Here's how the part is built. I have some questions about the finished solid (model axes, mm). A direction names the side the tool comes from. Coordinates: 2 decimals unless noted, no trailing zeros. Loops run counter-clockwise (first coordinate to the right, second up) from the corner with the lowest first, then second, coordinate; pieces in that order, holes last. Notation, with made-up numbers: M 58,53 L 65,53 A18 cw 65,76 Z; hole C 22,84 d4. An arc over 180 degrees is marked long. Use one line per item in the form item = value. Start each with the question number.
(1) On a 3-axis mill with a long thin cutter (end or side, diameter ignored), from which of +Z, -Z, +X, -X, +Y, -Y can I reach the whole of each face in a straight line? I mean faces 5 (the flat face through (2.87, -3, 5)), 6 (the flat face through (0, 0, 22)). Say none if no direction works.
(2) Imagine slicing it at C-C, the plane z = 30.5. Please give me the cut outline in (x, y), and give its area (3 significant figures).
(3) Thinking about a two-plate mould opening in Z: for faces 1 (the flat face through (0, -2, 45)), 2 (the flat face through (1.455, -2.837, 7.788)), 3 (the flat face through (0, -2, 0)), 4 (the flat face through (5.44, -1, 22)), which applies, +Z half, -Z half, draft (parallel to the pull), parting line (faces both ways), or undercut?
(4) Imagine slicing it at D-D, the plane x = 2. Please give me the cut outline in (y, z), and give its area (3 significant figures).
(5) Will these pins go through, and if not, where does the flat tip stop? P1, Ø1.9, axis at y = -3, z = 4.5, coming from the -X side; P2, Ø3, axis at x = -1, z = 5, coming from the -Y side; P3, Ø1.9, axis at y = -3, z = 40, coming from the +X side; P4, Ø1, axis at x = -1.5, y = -0.5, coming from the -Z side.
(6) Imagine slicing it at B-B, the plane y = -2.4. Please give me the cut outline in (x, z), and give its area (3 significant figures).
(7) Imagine slicing it at A-A, the plane x = -0.5. Please give me the cut outline in (y, z), and give its area (3 significant figures).
(8) Please list where these lines run through material, in increasing order: L1, parallel to Z at x = 0, y = -0.4; L2, parallel to Z at x = 1, y = -1.5 (3 decimals); L3, parallel to Y at x = 2, z = 39.
```python
from build123d import *

# Parameters (mm, degrees)
PAD_DEPTH       = 45
SKETCH001_R     = 1.6
POCKET_DEPTH    = 4.001
POCKET001_DEPTH = 2.36


with BuildPart() as part:
    # Sketch → Pad (new body)
    with BuildSketch(Plane.XY):
        Polygon((0, 0), (-5.44, 0), (-5.44, -1.68), (-2.94, -4), (0, -4), (2.94, -4), (5.44, -1.68), (5.44, 0), align=None)
    extrude(amount=PAD_DEPTH)

    # Sketch001 (on Face5 of Pad) → Pocket (cut, through all)
    with BuildSketch(Plane.XZ.offset(4)):
        with Locations((0, 39.686009)):
            Circle(SKETCH001_R)
        with Locations((0, 5.313991)):
            Circle(SKETCH001_R)
    extrude(amount=-POCKET_DEPTH, mode=Mode.SUBTRACT)

    # Sketch002 (on Face10 of Pocket) → Pocket001 (cut)
    with BuildSketch(Plane.XZ.offset(4)):
        Polygon((2.87, 41.343005), (0, 43), (-2.87, 41.343005), (-2.87, 38.029014), (0, 36.372019), (2.87, 38.029014), align=None)
        Polygon((2.87, 6.970986), (0, 8.627981), (-2.87, 6.970986), (-2.87, 3.656995), (0, 2), (2.87, 3.656995), align=None)
    extrude(amount=-POCKET001_DEPTH, mode=Mode.SUBTRACT)


solid = part.part
```
Answer:
q1.face_5 = -Y
q1.face_6 = +Z, -Z, +X, -X, +Y
q2.outline = M -5.44,-1.68 L -2.94,-4 L 2.94,-4 L 5.44,-1.68 L 5.44,0 L -5.44,0 Z
q2.area = 37.7 mm²
q3.face_1 = +Z half
q3.face_2 = undercut
q3.face_3 = -Z half
q3.face_4 = draft
q4.outline = M -4,0 L 0,0 L 0,45 L -4,45 L -4,41.85 L -1.64,41.85 L -1.64,37.53 L -4,37.53 L -4,7.47 L -1.64,7.47 L -1.64,3.15 L -4,3.15 Z
q4.area = 160 mm²
q5.P1 = -5.04
q5.P2 = -1.64
q5.P3 = 5.04
q5.P4 = 0
q6.outline = M -4.66,0 L 4.66,0 L 4.66,45 L -4.66,45 Z; hole M -2.87,3.66 L 0,2 L 2.87,3.66 L 2.87,6.97 L 0,8.63 L -2.87,6.97 Z; hole M -2.87,38.03 L 0,36.37 L 2.87,38.03 L 2.87,41.34 L 0,43 L -2.87,41.34 Z
q6.area = 363 mm²
q7.outline = M -4,0 L 0,0 L 0,3.79 L -1.64,3.79 L -1.64,2.29 L -4,2.29 Z; M -4,8.34 L -1.64,8.34 L -1.64,6.83 L 0,6.83 L 0,38.17 L -1.64,38.17 L -1.64,36.66 L -4,36.66 Z; M -4,42.71 L -1.64,42.71 L -1.64,41.21 L 0,41.21 L 0,45 L -4,45 Z
q7.area = 141 mm²
q8.L1 = 0 to 3.71, 6.91 to 38.09, 41.29 to 45
q8.L2 = 0 to 4.065, 6.563 to 38.437, 40.935 to 45
q8.L3 = -1.64 to 0
